```python
from build123d import *

# Parameters (mm, degrees)
F0_R     = 25
F1_DEPTH = 25
F2_T     = -5
F3_R     = 2.5
F4_R     = 2.5


with BuildPart() as f1:
    # F0 (on Top) → F1 (new body)
    with BuildSketch(Plane.XY):
        Circle(F0_R)
    extrude(amount=F1_DEPTH)

    # F2
    f2_openings = [f1.faces().sort_by_distance(p)[0] for p in [
        (0, 0, 0),
    ]]
    offset(amount=F2_T, openings=f2_openings)

    # F3
    f3_edges = [f1.edges().sort_by_distance(p)[0] for p in [
        (-25, 0, 25),
    ]]
    fillet(f3_edges, radius=F3_R)

    # F4
    f4_edges = [f1.edges().sort_by_distance(p)[0] for p in [
        (-25, 0, 0),
    ]]
    fillet(f4_edges, radius=F4_R)


solid = f1.part
```
Check sheet for the modelled part. Datum: model origin and axes. Units: mm. Round coordinates to 2 decimals unless told otherwise and drop trailing zeros. Write each loop counter-clockwise with the first axis right and the second up, starting at its lowest first coordinate (ties: lowest second). Pieces come first, ordered by that corner, then holes. Notation, with made-up numbers: (57, -10) -> (76, -10) arc R11 cw to (76, -4) -> close; hole circle Ø4 at (8, -10.75). An arc over 180 degrees is marked (long way). Put each result on its own line as item: value.
(1) Sectioned sample at C-C (z = 18.5). Enter the section's corners in (x, y).
Values found:
outline: circle Ø50 at (0, 0); hole circle Ø40 at (0, 0)
(2) Mould release check, pull along X, two halves, no side actions. Record for faces 1 (the face through (23.846, 7.509, 12.36)), 2 (the face through (-4.336, -19.524, 9.86)), 3 (the face through (0, 0, 20)), 4 (the face through (-20.1, -1.6, 0)): released by +X, released by -X, zero draft, split by the parting line, or undercut.
Values found:
face 1: split by the parting line
face 2: undercut
face 3: undercut
face 4: zero draft
(3) Material ranges on line 1 (Y direction, x = 0, z = 10.25); line 2 (Z direction, x = 8, y = -5); line 3 (Y direction, x = 1.5, z = 12.75), recorded low to high.
Values found:
line 1: y = -25 to -20, 20 to 25
line 2: z = 20 to 25
line 3: y = -24.95 to -19.94, 19.94 to 24.95
(4) Sectioned sample at A-A (y = 0). Enter the section's corners in (x, z).
Values found:
outline: (-25, 2.5) arc R2.5 ccw to (-22.5, 0) -> (-20, 0) -> (-20, 20) -> (20, 20) -> (20, 0) -> (22.5, 0) arc R2.5 ccw to (25, 2.5) -> (25, 22.5) arc R2.5 ccw to (22.5, 25) -> (-22.5, 25) arc R2.5 ccw to (-25, 22.5) -> close
(5) Go/stop test with flat-tipped pins: pin 1 Ø12 at (x, y) = (-9.5, -8.5) entering from -Z; pin 2 Ø1.5 at (y, z) = (1.5, 5) entering from +X; pin 3 Ø3 at (y, z) = (8, 13) entering from -X. Record where each tip stops, or that it passes through.
Values found:
pin 1: stops at z = 20
pin 2: stops at x = 24.99
pin 3: stops at x = -24.14
